Geometry: final body of the model. Coordinates: model frame, mm. Give positions to 0.01 mm unless a question says otherwise; leave off trailing zeros. Order: outer loops, then holes, each group sorted by start corner. A loop starts at its lowest first (then second) coordinate and runs counter-clockwise, first axis right, second up. Notation, with made-up numbers: (-28.75, 8.5) - (-15.75, 8.5) arc R16 ccw to (-15.75, 13.5) - close; hole circle Ø2 at (39.25, 27.25). An arc over 180 degrees is marked (long way). Write item = value, one per line. Start each with the question number.
from build123d import *

# Parameters (mm, degrees)
F0_W     = 736.6
F0_H     = 76.2
F1_DEPTH = 38.1
F2_SIZE  = 38.1
F3_W     = 76.2
F3_H     = 12.7
F4_DEPTH = 50.8


with BuildPart() as f1:
    # F0 (on Front) → F1 (new body)
    with BuildSketch(Plane.XZ):
        with Locations((0, 38.1)):
            Rectangle(F0_W, F0_H)
    extrude(amount=F1_DEPTH)

    # F2
    f2_edges = [f1.edges().sort_by_distance(p)[0] for p in [
        (-368.3, -19.05, 76.2),
        (368.3, -19.05, 76.2),
    ]]
    chamfer(f2_edges, length=F2_SIZE)

    # F3 (on face) → F4 (cut)
    with BuildSketch(Plane.XY.offset(76.2)):
        with Locations((-139.7, -19.05)):
            Rectangle(F3_W, F3_H)
        with Locations((139.7, -19.05)):
            Rectangle(F3_W, F3_H)
    extrude(amount=-F4_DEPTH, mode=Mode.SUBTRACT)


solid = f1.part
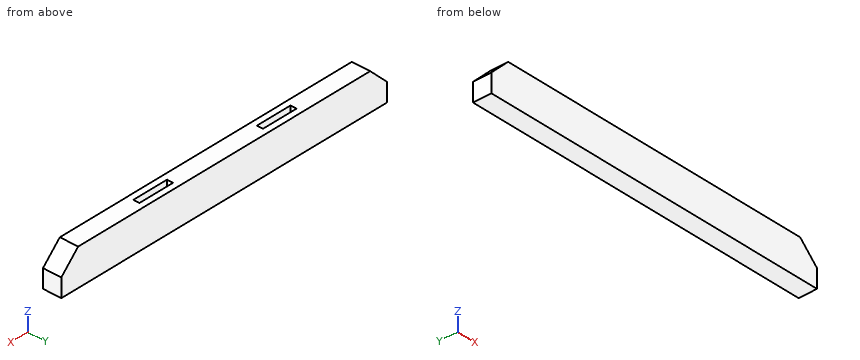
Q1. Section C-C, the plane y = -6.5. Return the cut outline in (x, z).
Q2. Section A-A, the plane z = 51.5. Return the cut outline in (x, y), then the cut area to 3 significant figures.
Q3. Section B-B, the plane x = -130. Return the cut outline in (y, z).
Q4. Contact query for flat-ended pins moving along their axis: pin 1 (3 mm diameter, centred on y = -22.5, z = 44.5, fed in from +X); pin 2 (4 mm diameter, centred on y = -17, z = 42.5, fed in from +X); pin 3 (6 mm diameter, centred on y = -27, z = 47, fed in from -X). Output: stop coordinate, or through.
Q5. Material intervals for line 1 along X through (y, z) = (-14, 37); line 2 along Y through (x, z) = (-155, 52); line 3 along X through (y, z) = (-13, 58), sorted ascending. Write a range as from..to.
The answers:
q1.outline = (-368.3, 0) - (368.3, 0) - (368.3, 38.1) - (330.2, 76.2) - (-330.2, 76.2) - (-368.3, 38.1) - close
q2.outline = (-354.9, -38.1) - (354.9, -38.1) - (354.9, 0) - (-354.9, 0) - close; hole (-177.8, -25.4) - (-101.6, -25.4) - (-101.6, -12.7) - (-177.8, -12.7) - close; hole (101.6, -25.4) - (177.8, -25.4) - (177.8, -12.7) - (101.6, -12.7) - close
q2.area = 25,100 mm²
q3.outline = (-38.1, 0) - (0, 0) - (0, 76.2) - (-12.7, 76.2) - (-12.7, 25.4) - (-25.4, 25.4) - (-25.4, 76.2) - (-38.1, 76.2) - close
q4.pin_1 = 363.4
q4.pin_2 = 365.9
q4.pin_3 = -362.4
q5.line_1 = -368.3..-177.8, -101.6..101.6, 177.8..368.3
q5.line_2 = -38.1..-25.4, -12.7..0
q5.line_3 = -348.4..-177.8, -101.6..101.6, 177.8..348.4
